from build123d import *

# Parameters (mm, degrees)
SKETCH_2_R       = 0.75
SKETCH_13_R      = 0.75
EXTRUDE_7_DEPTH  = 30
SKETCH_14_R      = 0.75
EXTRUDE_8_DEPTH  = 30
SKETCH_15_R      = 0.75
EXTRUDE_9_DEPTH  = 75
SKETCH_17_R      = 0.75
EXTRUDE_10_DEPTH = 10


with BuildPart() as part:
    # 扫描1: sweep along a path in 草图1
    with BuildLine(Plane.XY) as sweep_1_path:
        Line((50, 0), (50, 25))
        ThreePointArc((50, 25), (48.535533906, 28.535533906), (45, 30))
        Line((45, 30), (-80, 30))
        ThreePointArc((-80, 30), (-83.535533906, 28.535533906), (-85, 25))
        Line((-85, 25), (-85, 0))
    # 草图2 → 扫描1 (sweep)
    with BuildSketch(Plane(origin=(0, 0, 0), x_dir=(1, 0, 0), z_dir=(0, 1, 0))):
        with Locations((-85, 0)):
            Circle(SKETCH_2_R)
    sweep(path=sweep_1_path.line)

    # 草图13 → 凸台-拉伸7 (add)
    with BuildSketch(Plane(origin=(0, 0, 0), x_dir=(1, 0, 0), z_dir=(0, 1, 0))):
        with Locations((40, 0)):
            Circle(SKETCH_13_R)
    extrude(amount=EXTRUDE_7_DEPTH)

    # 草图14 → 凸台-拉伸8 (add)
    with BuildSketch(Plane(origin=(0, 0, 0), x_dir=(-1, 0, 0), z_dir=(0, 1, 0))):
        with Locations((10, 0)):
            Circle(SKETCH_14_R)
    extrude(amount=EXTRUDE_8_DEPTH)

    # 草图15 → 凸台-拉伸9 (add)
    with BuildSketch(Plane(origin=(-85, 0, 0), x_dir=(0, 0, -1), z_dir=(1, 0, 0))):
        with Locations((0, 15)):
            Circle(SKETCH_15_R)
    extrude(amount=EXTRUDE_9_DEPTH)

    # 草图17 → 凸台-拉伸10 (add)
    with BuildSketch(Plane(origin=(50, 15, 0), x_dir=(0, 0, 1), z_dir=(-1, 0, 0))):
        Circle(SKETCH_17_R)
    extrude(amount=EXTRUDE_10_DEPTH)


solid = part.part
Work out the finished part from the listing and answer in its coordinate system (mm). Give positions to 0.01 mm unless a question says otherwise; leave off trailing zeros. Order: outer loops, then holes, each group sorted by start corner. A loop starts at its lowest first (then second) coordinate and runs counter-clockwise, first axis right, second up. Notation, with made-up numbers: (32, -27) -> (38, -27) arc R29 cw to (38, 0) -> close; hole circle Ø1 at (8, -6). An arc over 180 degrees is marked (long way). One line per item, written item: value.
Item 1: Find section A-A, the plane z = 0. Give the vertices of the cut face in (x, y).
Answer sheet:
outline: (-85.75, 0) -> (-84.25, 0) -> (-84.25, 14.25) -> (-10.75, 14.25) -> (-10.75, 0) -> (-9.25, 0) -> (-9.25, 29.25) -> (39.25, 29.25) -> (39.25, 0) -> (40.75, 0) -> (40.75, 14.25) -> (49.25, 14.25) -> (49.25, 0) -> (50.75, 0) -> (50.75, 25) arc R5.75 ccw to (45, 30.75) -> (-80, 30.75) arc R5.75 ccw to (-85.75, 25) -> close; hole (-84.25, 15.75) -> (-10.75, 15.75) -> (-10.75, 29.25) -> (-80, 29.25) arc R4.25 ccw to (-84.25, 25) -> close; hole (40.75, 15.75) -> (49.25, 15.75) -> (49.25, 25) arc R4.25 ccw to (45, 29.25) -> (40.75, 29.25) -> close
Item 2: A flat-ended cylindrical pin translates along its axis: P1, Ø8, axis at x = 14.5, y = 25, coming from the +Z side. Find the tip coordinate at first contact, or state that the pin passes through.
Answer sheet:
P1: through
Item 3: Find section D-D, the plane x = 21.5. Give the vertices of the cut face in (y, z).
Answer sheet:
outline: circle Ø1.5 at (30, 0)
Item 4: Find section C-C, the plane y = 22.5. Give the vertices of the cut face in (x, z), plus the area to 3 significant figures.
Answer sheet:
outline: circle Ø1.5 at (-85, 0); circle Ø1.5 at (-10, 0); circle Ø1.5 at (40, 0); circle Ø1.5 at (50, 0)
area: 7.07 mm²
Item 5: Straight lines are drawn through the part: probe 1 along X at (y, z) = (3, -0.2); probe 2 along Y at (x, z) = (-26.5, -0.1); probe 3 along X at (y, z) = (12, -0.6). For each, find the intervals that lie inside material, in ascending order.
Answer sheet:
probe 1: -85.72 to -84.28, -10.72 to -9.28, 39.28 to 40.72, 49.28 to 50.72
probe 2: 14.26 to 15.74, 29.26 to 30.74
probe 3: -85.45 to -84.55, -10.45 to -9.55, 39.55 to 40.45, 49.55 to 50.45
Item 6: Find section B-B, the plane x = -75.5. Give the vertices of the cut face in (y, z).
Answer sheet:
outline: circle Ø1.5 at (15, 0); circle Ø1.5 at (30, 0)
